from build123d import *

# Parameters (mm, degrees)
BOSS_EXTRUDE1_DEPTH = 6.35
FILLET1_R           = 2.54
SKETCH2_W           = 3.39204747
SKETCH2_H           = 4.630409642
CUT_EXTRUDE1_DEPTH  = 57.994566408
FILLET2_R           = 1.27


with BuildPart() as part:
    # Sketch1 → Boss-Extrude1 (new body)
    with BuildSketch(Plane(origin=(0, 0, 0), x_dir=(1, 0, 0), z_dir=(0, 1, 0))):
        with BuildLine():
            Line((0, 0), (16.51, 0))
            ThreePointArc((16.51, 0), (18.306051224, 0.743948776), (19.05, 2.54))
            Line((19.05, 2.54), (19.05, 8.89))
            Line((19.05, 8.89), (38.1, 8.89))
            ThreePointArc((38.1, 8.89), (19.05, 27.94), (38.1, 46.99))
            Line((38.1, 46.99), (19.05, 46.99))
            Line((19.05, 46.99), (19.05, 53.34))
            Line((19.05, 53.34), (18.415, 53.34))
            ThreePointArc((18.415, 53.34), (16.618948776, 52.596051224), (15.875, 50.8))
            Line((15.875, 50.8), (15.875, 15.875))
            ThreePointArc((15.875, 15.875), (12.155256121, 6.894743879), (3.175, 3.175))
            Line((3.175, 3.175), (2.54, 3.175))
            ThreePointArc((2.54, 3.175), (0.743948776, 2.431051224), (0, 0.635))
            Line((0, 0.635), (0, 0))
        make_face()
        Polygon((24.973677906, 10.795), (17.78, 19.806028114), (17.78, 10.795), align=None, mode=Mode.SUBTRACT)
        Polygon((17.78, 45.085), (24.973677906, 45.085), (17.78, 36.073971886), align=None, mode=Mode.SUBTRACT)
    extrude(amount=BOSS_EXTRUDE1_DEPTH)

    # Fillet1
    fillet1_edges = [part.edges().sort_by_distance(p)[0] for p in [
        (38.1, 3.175, -46.99),
        (38.1, 3.175, -8.89),
    ]]
    fillet(fillet1_edges, radius=FILLET1_R)

    # Sketch2 → Cut-Extrude1 (cut, through all)
    with BuildSketch(Plane(origin=(19.05, 0, 0), x_dir=(0, 0, -1), z_dir=(1, 0, 0))):
        with Locations((7.193976265, 3.175)):
            Rectangle(SKETCH2_W, SKETCH2_H)
        with Locations((48.686023735, 3.175)):
            Rectangle(SKETCH2_W, SKETCH2_H)
    extrude(amount=-CUT_EXTRUDE1_DEPTH, mode=Mode.SUBTRACT)

    # Fillet2
    fillet2_edges = [part.edges().sort_by_distance(p)[0] for p in [
        (17.78, 3.175, -10.795),
        (24.973677906, 3.175, -10.795),
        (17.78, 3.175, -19.806028114),
        (17.78, 3.175, -36.073971886),
        (24.973677906, 3.175, -45.085),
        (17.78, 3.175, -45.085),
        (13.781591111, 3.175, -8.89),
        (15.875, 3.175, -46.99),
    ]]
    fillet(fillet2_edges, radius=FILLET2_R)


solid = part.part
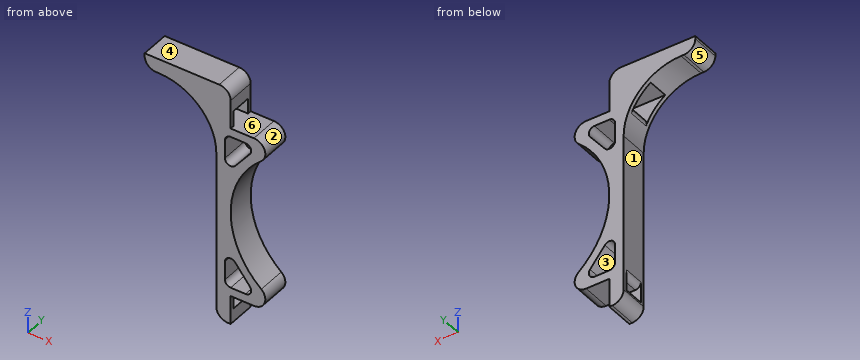
Design review of the part built by this model. Coordinates are the model's own, in mm. Face numbers are marked on the shaded views. A direction names the side the tool comes from. Round coordinates to 2 decimals unless told otherwise and drop trailing zeros. Write each loop counter-clockwise with the first axis right and the second up, starting at its lowest first coordinate (ties: lowest second). Pieces come first, ordered by that corner, then holes. Notation, with made-up numbers: (39.25, 13) -> (97.25, 13) arc R8 cw to (97.25, 21) -> close; hole circle Ø7 at (80.25, 31). An arc over 180 degrees is marked (long way). One line per item, written item: value. Start each with the question number.
Q1. To check wall thickness, follow probe 1 along Z at (x, y) = (22.25, 4.5) (3 decimals); probe 2 along Z at (x, y) = (18.25, 1.5); probe 3 along Z at (x, y) = (17, 1). State the ranges of each line that lie inside material, in increasing order.
Q2. Add section D-D (z = -34). Give the boundary of the cut face in (x, y) (3 decimals).
Q3. The part is to be moulded in two halves that separate along Z. For the marked faces 3, 4, 5 and 6, say which applies: pulls with the +Z half, pulls with the -Z half, needs draft (parallel to the pull), parting line crosses it, or undercut.
Q4. Add section B-B (z = -14). Give the boundary of the cut face in (x, y), then the cut area to 3 significant figures.
Q5. Insertion check: P1, Ø1.5, axis at y = 1, z = -26.5, coming from the +X side; P2, Ø1.9, axis at y = 4, z = -6, coming from the +X side; P3, Ø2, axis at y = 1, z = -36, coming from the +X side. Each pin has a flat end and moves straight along its axis. Give the tip position at first contact, or say it passes through.
Q6. Add section C-C (x = 12). Give the boundary of the cut face in (y, z), then the cut area to 3 significant figures.
Q7. Tool access review of the marked faces 1 and 2: name each direction out of +Z, -Z, +X, -X, +Y, -Y from which nothing blocks a thin tool from reaching the whole face with its end or side.
Q8. Add section A-A (y = 2). State how many separate pieces and enclosed holes the cut face has, then the cut area to 3 significant figures.
Response:
1. probe 1: z = -46.99 to -45.085, -41.673 to -38.508, -17.372 to -14.207, -10.795 to -8.89
1. probe 2: z = -53.33 to -50.38, -46.99 to -44.8, -38.71 to -17.17, -11.08 to -8.89, -5.5 to -0.69
1. probe 3: z = -52.91 to -50.38, -46.98 to -8.89, -5.5 to -0.05
2. outline: (15.875, 0) -> (20.04, 0) -> (20.04, 6.35) -> (15.875, 6.35) -> close
3. face 3: undercut
3. face 4: pulls with the +Z half
3. face 5: pulls with the -Z half
3. face 6: undercut
4. outline: (15.74, 0) -> (17.78, 0) -> (17.78, 6.35) -> (15.74, 6.35) -> close; (22.42, 0) -> (25.12, 0) -> (25.12, 6.35) -> (22.42, 6.35) -> close
4. area: 30.1 mm^2
5. P1: stops at x = 19.18
5. P2: stops at x = 19.05
5. P3: stops at x = 21.34
6. outline: (0, -6.74) -> (0.86, -6.74) -> (0.86, -5.5) -> (5.49, -5.5) -> (5.49, -6.74) -> (6.35, -6.74) -> (6.35, 0) -> (0, 0) -> close
6. area: 37.1 mm^2
7. face 1: -Z, -X, +Y, -Y
7. face 2: +X, +Y, -Y
8. separate pieces: 3
8. enclosed holes: 2
8. area: 285 mm^2
